The listing builds one solid part. Answer for the finished solid, in the listing's coordinates (mm). Face numbers are marked on the shaded views. A direction names the side the tool comes from. Round coordinates to 2 decimals unless told otherwise and drop trailing zeros. Write each loop counter-clockwise with the first axis right and the second up, starting at its lowest first coordinate (ties: lowest second). Pieces come first, ordered by that corner, then holes.
Item 1: Each of these flat-tipped pins is pushed along its axis until it touches: pin 1 (19.5 mm diameter, centred on x = -16.5, y = 3, fed in from +Z); pin 2 (10 mm diameter, centred on x = -5.5, z = 43, fed in from +Y); pin 3 (0.6 mm diameter, centred on x = 0, z = 55.5, fed in from -Y); pin 4 (3.5 mm diameter, centred on x = 23, y = 0, fed in from -Z). Where does it stop, or does it pass through?
Item 2: Find section C-C on y = 0. Give the number of separate pieces and of enclosed holes in the cut face, then the cut area to 3 significant figures.
Item 3: For a pull along Z with two mould halves and no side action, classify the marked faces 5, 6 and 7 as +Z half, -Z half, draft (parallel to the pull), parting line (faces both ways), or undercut.
Item 4: A tool of negligible diameter and unlimited length cuts with its end or side. For the marked faces 1, 2, 3 and 4, from which of +Z, -Z, +X, -X, +Y, -Y can it reach the whole face along a straight path? Write none if from no direction.
Item 5: Find the intervals of material crossed by probe 1 along Z at (x, y) = (-2, -11.5); probe 2 along Z at (x, y) = (19, 1.5); probe 3 along Z at (x, y) = (9, 10), in increasing order.
Item 6: Find section D-D on x = 0. Give the vertices of the cut face in (y, z).
Item 7: Find section B-B on x = 23. Give the vertices of the cut face in (y, z).
Item 8: Find section A-A on z = 8. Give the vertices of the cut face in (x, y), then the cut area to 3 significant figures.
Autodesk Inventor part; units mm, degrees
ref_plane "YZ Plane" through (0, 0, 0) normal (1, 0, 0) x (0, 1, 0)
ref_plane "XZ Plane" through (0, 0, 0) normal (0, 1, 0) x (-1, 0, 0)
ref_plane "XY Plane" through (0, 0, 0) normal (0, 0, 1) x (1, 0, 0)
sketch "Base" plane through (0, 0, 0) normal (0, 0, 1) x (1, 0, 0)
  circle A0 centre (0, 0) radius 17.5
  circle A1 centre (23, 0) radius 2.25
  line L0 (-38.5, 0) -> (38.5, 0) construction
  line L1 (0, -24.5) -> (0, 24.5) construction
  circle A2 centre (-23, 0) radius 2.25
  circle A3 centre (23, 0) radius 4.5
  circle A4 centre (-23, 0) radius 4.5
  line L2 (-27.5, 0) -> (27.5, 0) construction
  line L3 (9.8913, 14.4365) -> (25.5435, 3.7122)
  line L4 (25.5435, -3.7122) -> (9.8913, -14.4365)
  line L5 (-25.5435, 3.7122) -> (-9.8913, 14.4365)
  line L6 (-25.5435, -3.7122) -> (-9.8913, -14.4365)
  dimension "d0" = 35
  dimension "d1" = 4.5
  dimension "d2" = 2.25
  dimension "d3" = 46
  dimension "d4" = 55
extrude "BaseFeature" add sketch "Base" along normal blind 10
sketch "Body" plane through (0, 0, 10) normal (0, 0, 1) x (1, 0, 0)
  circle A0 centre (0, 0) radius 17.5
  arc A1 (-9.8913, -14.4365) -> (9.8913, -14.4365) centre (0, 0) ccw
extrude "BodyFeature" add sketch "Body" along normal blind 28
sketch "Head" plane through (0, 0, 38) normal (0, 0, 1) x (1, 0, 0)
  circle A0 centre (0, 0) radius 20
  dimension "d9" = 40
extrude "HeadFeature" add sketch "Head" along normal blind 11.5
sketch "Top" plane through (0, 0, 49.5) normal (0, 0, 1) x (1, 0, 0)
  circle A0 centre (0, 0) radius 18.2
  circle A1 centre (0, 0) radius 20
  dimension "d12" = 1.8
extrude "TopFeature" cut sketch "Top" against normal blind 0.5 contours A0
sketch "Sketch5" plane through (0, 0, 49) normal (0, 0, 1) x (1, 0, 0)
  line L0 (-38.5, 0) -> (38.5, 0) construction
  circle A0 centre (8.8, 0) radius 4.7
  line L1 (0, -28) -> (0, 28) construction
  circle A1 centre (-8.8, 0) radius 4.7
  line L2 (8.8, 0) -> (13.5, 0) construction
  line L3 (-8.8, 0) -> (-13.5, 0) construction
  point P0 (0, 0)
  dimension "d15" = 9.4
  dimension "d16" = 27
extrude "Extrusion5" add sketch "Sketch5" along normal blind 3
sketch "Sketch6" plane through (8.8, 0, 52) normal (0, 0, 1) x (1, 0, 0)
  circle A0 centre (0, 0) radius 4.7
  circle A1 centre (-17.6, 0) radius 4.7
  circle A2 centre (-17.6, 0) radius 4.7
  circle A3 centre (-17.6, 0) radius 2.15
  circle A4 centre (0, 0) radius 2.15
  point P0 (-8.8, 0)
  dimension "d19" = 4.3
extrude "Extrusion6" cut sketch "Sketch6" against normal blind 6 contours A3 | A4
sketch "Sketch7" plane through (0, 0, 49) normal (0, 0, 1) x (1, 0, 0)
  circle A0 centre (-8.8, 0) radius 4.7
  circle A1 centre (8.8, 0) radius 4.7
  circle A2 centre (0, 0) radius 18.2
  line L0 (-18.2, 1.625) -> (18.2, 1.625)
  line L1 (18.2, 1.625) -> (18.2, -1.625)
  line L2 (18.2, -1.625) -> (-18.2, -1.625)
  line L3 (-18.2, -1.625) -> (-18.2, 1.625)
  line L4 (-38.5, 0) -> (38.5, 0) construction
  circle A3 centre (0, 0) radius 18.2
  point P0 (-18.2, 0)
  point P1 (13.2101, -1.625)
  point P2 (18.1273, -1.625)
  point P3 (18.1273, 1.625)
  point P4 (13.2101, 1.625)
  point P5 (-4.3899, -1.625)
  point P6 (4.3899, -1.625)
  point P7 (4.3899, 1.625)
  point P8 (-4.3899, 1.625)
  point P9 (-18.1273, -1.625)
  point P10 (-13.2101, -1.625)
  point P11 (-13.2101, 1.625)
  point P12 (-18.1273, 1.625)
  dimension "d22" = 3.25
extrude "Extrusion7" add sketch "Sketch7" along normal up to surface (0.5 mm away) contours A0 L0 A1 L2 | A0 L2 A2 L0 | L0 A2 L2 A1
sketch "Sketch8" plane through (0, 0, 49) normal (0, 0, 1) x (1, 0, 0)
  line L0 (0, -28) -> (0, 28) construction
  line L1 (-1, 18.2) -> (1, 18.2)
  line L2 (1, 18.2) -> (1, -18.2)
  line L3 (1, -18.2) -> (-1, -18.2)
  line L4 (-1, -18.2) -> (-1, 18.2)
  arc A0 (18.1273, 1.625) -> (-18.1273, 1.625) centre (0, 0) ccw
  arc A1 (-18.1273, -1.625) -> (18.1273, -1.625) centre (0, 0) ccw
  point P0 (0, 18.2)
  dimension "d25" = 2
extrude "Extrusion8" add sketch "Sketch8" along normal up to surface (0.5 mm away)
sketch "Sketch9" plane through (0, 0, 49.5) normal (0, 0, 1) x (1, 0, 0)
  line L0 (0, -28) -> (0, 28) construction
  circle A0 centre (0, -12.8363) radius 2.5
  line L1 (-1, 1.625) -> (-1, 18.1725)
  line L2 (1, -1.625) -> (1, -18.1725)
  line L3 (-1, 7.5) -> (1, 7.5)
  line L4 (1, 7.5) -> (1, -7.5)
  line L5 (1, -7.5) -> (-1, -7.5)
  line L6 (-1, -7.5) -> (-1, 7.5)
  line L7 (-38.5, 0) -> (38.5, 0) construction
  line L8 (0, -7.5) -> (0, -18.1725) construction
  point P0 (0, 0)
  point P1 (1, 0)
  dimension "d28" = 5
  dimension "d29" = 15
  dimension "d30" = 5.3362
  dimension "d31" = 5.3362
extrude "Extrusion9" add sketch "Sketch9" along normal blind 9
equation "\"d26\" = d25"
properties part number "HiitioContactor"
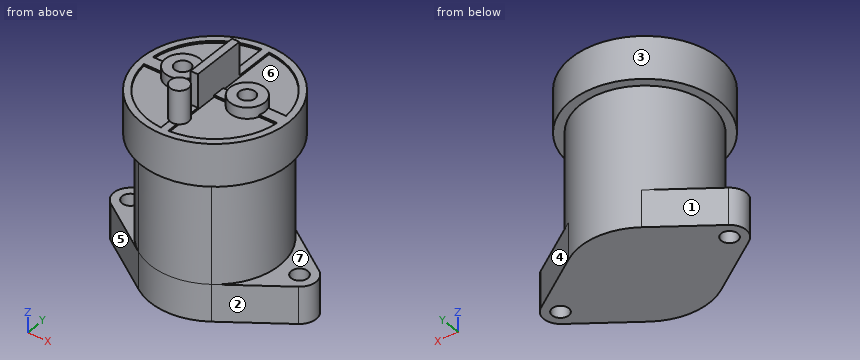
Check values:
1. pin 1: stops at z = 52
1. pin 2: stops at y = 19.99
1. pin 3: stops at y = -15.34
1. pin 4: passes through
2. separate pieces: 3
2. enclosed holes: 0
2. area: 1,910 mm2
3. face 5: draft
3. face 6: +Z half
3. face 7: undercut
4. face 1: -Z, -X, +Y
4. face 2: -Z, +X, -Y
4. face 3: +Z
4. face 4: -Z, +X, +Y
5. probe 1: z = 0 to 49, 49.5 to 58.5
5. probe 2: z = 0 to 10, 38 to 49.5
5. probe 3: z = 0 to 49
6. outline: (-20, 38) - (-17.5, 38) - (-17.5, 0) - (17.5, 0) - (17.5, 38) - (20, 38) - (20, 49.5) - (7.5, 49.5) - (7.5, 58.5) - (-7.5, 58.5) - (-7.5, 49.5) - (-10.34, 49.5) - (-10.34, 58.5) - (-15.34, 58.5) - (-15.34, 49.5) - (-20, 49.5) - close
7. outline: (-5.45, 0) - (-2.25, 0) - (-2.25, 10) - (-5.45, 10) - close; (2.25, 0) - (5.45, 0) - (5.45, 10) - (2.25, 10) - close
8. outline: (-25.54, -3.71) - (-9.89, -14.44) arc R17.5 ccw to (9.89, -14.44) - (25.54, -3.71) arc R4.5 ccw to (25.54, 3.71) - (9.89, 14.44) arc R17.5 ccw to (-9.89, 14.44) - (-25.54, 3.71) arc R4.5 ccw to start; hole circle Ø4.5 at (-23, 0); hole circle Ø4.5 at (23, 0)
8. area: 1,210 mm2
